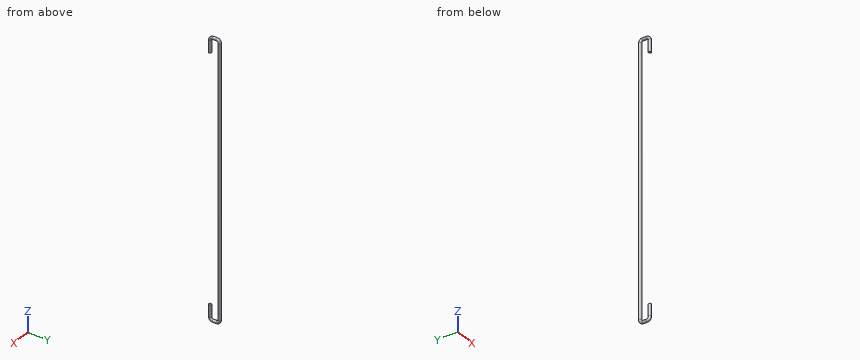
Autodesk Inventor part; units mm, degrees
ref_plane "YZ Plane" through (0, 0, 0) normal (1, 0, 0) x (0, 1, 0)
ref_plane "XZ Plane" through (0, 0, 0) normal (0, 1, 0) x (-1, 0, 0)
ref_plane "XY Plane" through (0, 0, 0) normal (0, 0, 1) x (1, 0, 0)
sketch "Sketch1" plane through (0, 0, 0) normal (0, 0, 1) x (1, 0, 0)
  circle A0 centre (0, 0) radius 0.5969
  dimension "d0" = 1.1938
sketch "Sketch2" plane through (0, 0, 0) normal (1, 0, 0) x (0, 1, 0)
  line L0 (0, 0) -> (0, 5.08)
  line L1 (1.27, 6.35) -> (2.8575, 6.35)
  line L2 (4.1275, 5.08) -> (4.1275, -107.95)
  line L3 (0, -107.95) -> (0, -102.87)
  line L4 (2.8575, -109.22) -> (1.27, -109.22)
  arc A0 (4.1275, 5.08) -> (2.8575, 6.35) centre (2.8575, 5.08) ccw
  arc A1 (2.8575, -109.22) -> (4.1275, -107.95) centre (2.8575, -107.95) ccw
  arc A2 (0, -107.95) -> (1.27, -109.22) centre (1.27, -107.95) ccw
  arc A3 (1.27, 6.35) -> (0, 5.08) centre (1.27, 5.08) ccw
  dimension "d1" = 1.27
  dimension "d5" = 1.5875
  dimension "d7" = 115.57
  dimension "d8" = 6.35
sweep "Sweep1" add profiles "Sketch1" path "Sketch2"
properties part number "Rudder_Link"
The listing builds one solid part. Answer for the finished solid, in the listing's coordinates (mm). Give positions to 0.01 mm unless a question says otherwise; leave off trailing zeros. Order: outer loops, then holes, each group sorted by start corner. A loop starts at its lowest first (then second) coordinate and runs counter-clockwise, first axis right, second up.
Item 1: Given pin 1 Ø3 at (y, z) = (1.5, -23.5) entering from -X, flat-ended and moving along its own axis, determine where the tip first touches the part or whether it passes through.
From the geometry:
pin 1: passes through
Item 2: The part is cut by section A-A, the plane x = 0. Give the vertices of the cut face in (y, z).
From the geometry:
outline: (-0.6, -107.95) arc R1.87 ccw to (1.27, -109.82) - (2.86, -109.82) arc R1.87 ccw to (4.72, -107.95) - (4.72, 5.08) arc R1.87 ccw to (2.86, 6.95) - (1.27, 6.95) arc R1.87 ccw to (-0.6, 5.08) - (-0.6, 0) - (0.6, 0) - (0.6, 5.08) arc R0.67 cw to (1.27, 5.75) - (2.86, 5.75) arc R0.67 cw to (3.53, 5.08) - (3.53, -107.95) arc R0.67 cw to (2.86, -108.62) - (1.27, -108.62) arc R0.67 cw to (0.6, -107.95) - (0.6, -102.87) - (-0.6, -102.87) - close
Item 3: Find the intervals of material crossed by probe 1 along Y at (x, z) = (0.1, -30.5); probe 2 along Z at (x, y) = (0.25, 3.15); probe 3 along Z at (x, y) = (-0.2, 1.25), in increasing order.
From the geometry:
probe 1: y = 3.54 to 4.72
probe 2: z = -109.74 to -108.62, 5.75 to 6.87
probe 3: z = -109.78 to -108.66, 5.79 to 6.91
Item 4: The part is cut by section B-B, the plane z = -90. Give the vertices of the cut face in (x, y), and give its area (3 significant figures).
From the geometry:
outline: circle Ø1.19 at (0, 4.13)
area: 1.12 mm2
